Work out the finished part from the listing and answer in its coordinate system (mm). A direction names the side the tool comes from. Coordinates: 2 decimals unless noted, no trailing zeros. Order: outer loops, then holes, each group sorted by start corner. A loop starts at its lowest first (then second) coordinate and runs counter-clockwise, first axis right, second up. Notation, with made-up numbers: (58, -40) - (89, -40) arc R21 cw to (89, -13) - close; hole circle Ø2 at (18, 67.5). An arc over 180 degrees is marked (long way). Answer as a JSON object with one key per item and string values. Group by question number.
1) A tool of negligible diameter and unlimited length cuts with its end or side. For faces 1 (the face through (-33, -17, 10)), 2 (the face through (0, 22, 10)), 3 (the face through (-36, -22, 10)), 4 (the face through (-47.5, 0, 10)), from which of +Z, -Z, +X, -X, +Y, -Y can it reach the whole face along a straight path? Write none if from no direction.
2) Section A-A (x = 53.8) is taken. Give the vertices of the cut face in (y, z).
3) The mould has two halves that part along Y. Classify faces 5 (the face through (13.5, 31.07, 2.54)), 6 (the face through (59, -35, 3)), 7 (the face through (-61, 0, 2)): released by +Y, released by -Y, zero draft, split by the parting line, or undercut.
4) Section D-D (x = -34) is taken. Give the vertices of the cut face in (y, z).
5) Each of these flat-tipped pins is pushed along its axis until it touches: P1, Ø4, axis at x = -15, y = 31, coming from the +Z side; P2, Ø6, axis at x = 45, z = 13, coming from the +Y side; P3, Ø8, axis at x = -33, z = 10, coming from the -Y side. Where does it stop, or does it pass through?
6) Find the intervals of material crossed by line 1 along Y through (x, z) = (-53.8, 2.7); line 2 along Y through (x, z) = (-17, 11.25); line 3 along Y through (x, z) = (-31, 6.5), in increasing order.
7) Section C-C (y = 12) is taken. Give the vertices of the cut face in (x, z).
8) Section B-B (x = -15) is taken. Give the vertices of the cut face in (y, z).
from build123d import *

# Parameters (mm, degrees)
SKETCH_1_W          = 122
SKETCH_1_H          = 72
EXTRUDE_1_DEPTH     = 5
SKETCH_4_R          = 1.5
CUT_EXTRUDE_2_DEPTH = 10
SKETCH_5_W          = 5
SKETCH_5_H          = 5
EXTRUDE_3_DEPTH     = 10
SKETCH_6_R          = 1.5
CUT_EXTRUDE_3_DEPTH = 15
CUT_EXTRUDE_4_DEPTH = 25
FILLET_1_R          = 4
FILLET_3_R          = 5


with BuildPart() as part:
    # 草图1 → 凸台-拉伸1 (new body)
    with BuildSketch(Plane.XY):
        Rectangle(SKETCH_1_W, SKETCH_1_H)
    extrude(amount=EXTRUDE_1_DEPTH)

    # 草图4 → 切除-拉伸2 (cut)
    with BuildSketch(Plane.XY.offset(5)):
        with Locations((-53.8, 12)):
            Circle(SKETCH_4_R)
        with Locations((53.8, 12)):
            Circle(SKETCH_4_R)
        with Locations((53.8, -12)):
            Circle(SKETCH_4_R)
        with Locations(Location((-53.8, -12, 0), (0, 0, 180))):
            Circle(SKETCH_4_R)
    extrude(amount=-CUT_EXTRUDE_2_DEPTH, mode=Mode.SUBTRACT)

    # 草图5 → 凸台-拉伸3 (add)
    with BuildSketch(Plane.XY.offset(5)):
        Polygon((-42.5, 17), (42.5, 17), (42.5, 22), (-47.5, 22), (-47.5, -22), (-25, -22), (-25, -17), (-42.5, -17), align=None)
        with Locations((-22.5, -19.5)):
            Rectangle(SKETCH_5_W, SKETCH_5_H)
        Polygon((25, -36), (25, -31), (20, -31), (-20, -31), (-20, -22), (-25, -22), (-25, -36), align=None)
    extrude(amount=EXTRUDE_3_DEPTH)

    # 草图6 → 切除-拉伸3 (cut)
    with BuildSketch(Plane.XY.offset(5)):
        with Locations((0, 31)):
            Circle(SKETCH_6_R)
        with Locations((15, 31)):
            Circle(SKETCH_6_R)
        with Locations((30, 31)):
            Circle(SKETCH_6_R)
        with Locations((-15, 31)):
            Circle(SKETCH_6_R)
        with Locations((-30, 31)):
            Circle(SKETCH_6_R)
    extrude(amount=-CUT_EXTRUDE_3_DEPTH, mode=Mode.SUBTRACT)

    # 草图7 → 切除-拉伸4 (cut)
    with BuildSketch(Plane.XY.offset(5)):
        with BuildLine():
            ThreePointArc((44.8, 31.8), (43.3, 33.3), (41.8, 31.8))
            Line((41.8, 31.8), (43.3, 31.8))
            Line((43.3, 31.8), (43.3, 30.3))
            ThreePointArc((43.3, 30.3), (44.360660172, 30.739339828), (44.8, 31.8))
        make_face()
        with BuildLine():
            Line((43.3, 31.8), (41.8, 31.8))
            ThreePointArc((41.8, 31.8), (42.239339828, 30.739339828), (43.3, 30.3))
            Line((43.3, 30.3), (43.3, 31.8))
        make_face()
        with BuildLine():
            ThreePointArc((44.8, -31.8), (44.360660172, -30.739339828), (43.3, -30.3))
            Line((43.3, -30.3), (43.3, -31.8))
            Line((43.3, -31.8), (41.8, -31.8))
            ThreePointArc((41.8, -31.8), (43.3, -33.3), (44.8, -31.8))
        make_face()
        with BuildLine():
            Line((43.3, -31.8), (43.3, -30.3))
            ThreePointArc((43.3, -30.3), (42.239339828, -30.739339828), (41.8, -31.8))
            Line((41.8, -31.8), (43.3, -31.8))
        make_face()
        with BuildLine():
            ThreePointArc((-41.8, -31.8), (-42.239339828, -30.739339828), (-43.3, -30.3))
            Line((-43.3, -30.3), (-43.3, -31.8))
            Line((-43.3, -31.8), (-41.8, -31.8))
        make_face()
        with BuildLine():
            Line((-43.3, -31.8), (-43.3, -30.3))
            ThreePointArc((-43.3, -30.3), (-44.360660172, -32.860660172), (-41.8, -31.8))
            Line((-41.8, -31.8), (-43.3, -31.8))
        make_face()
        with BuildLine():
            Line((-43.3, 30.3), (-43.3, 31.8))
            Line((-43.3, 31.8), (-41.8, 31.8))
            ThreePointArc((-41.8, 31.8), (-44.360660172, 32.860660172), (-43.3, 30.3))
        make_face()
        with BuildLine():
            Line((-41.8, 31.8), (-43.3, 31.8))
            Line((-43.3, 31.8), (-43.3, 30.3))
            ThreePointArc((-43.3, 30.3), (-42.239339828, 30.739339828), (-41.8, 31.8))
        make_face()
    extrude(amount=-CUT_EXTRUDE_4_DEPTH, mode=Mode.SUBTRACT)

    # 圆角1
    fillet_1_edges = [part.edges().sort_by_distance(p)[0] for p in [
        (-47.5, 22, 10),
        (-47.5, -22, 10),
        (-25, -22, 10),
        (-25, -36, 10),
        (-20, -17, 10),
    ]]
    fillet(fillet_1_edges, radius=FILLET_1_R)

    # 圆角3
    fillet_3_edges = [part.edges().sort_by_distance(p)[0] for p in [
        (61, -36, 2.5),
        (-61, -36, 2.5),
        (-61, 36, 2.5),
        (61, 36, 2.5),
    ]]
    fillet(fillet_3_edges, radius=FILLET_3_R)


solid = part.part
Report:
{
 "1": {"face 1": "+Z, +X", "face 2": "+Z, +X, -X, +Y", "face 3": "+Z, -X, -Y", "face 4": "+Z, -X, +Y, -Y"},
 "2": {"outline": "(-36, 0) - (-13.5, 0) - (-13.5, 5) - (-36, 5) - close; (-10.5, 0) - (10.5, 0) - (10.5, 5) - (-10.5, 5) - close; (13.5, 0) - (36, 0) - (36, 5) - (13.5, 5) - close"},
 "3": {"face 5": "undercut", "face 6": "released by -Y", "face 7": "zero draft"},
 "4": {"outline": "(-36, 0) - (36, 0) - (36, 5) - (22, 5) - (22, 15) - (17, 15) - (17, 5) - (-17, 5) - (-17, 15) - (-22, 15) - (-22, 5) - (-36, 5) - close"},
 "5": {"P1": "stops at z = 5", "P2": "stops at y = 22", "P3": "stops at y = -22"},
 "6": {"line 1": "y = -36 to -13.5, -10.5 to 10.5, 13.5 to 36", "line 2": "y = -36 to -31, 17 to 22", "line 3": "y = -22 to -17, 17 to 22"},
 "7": {"outline": "(-61, 0) - (-55.3, 0) - (-55.3, 5) - (-61, 5) - close; (-52.3, 0) - (52.3, 0) - (52.3, 5) - (-42.5, 5) - (-42.5, 15) - (-47.5, 15) - (-47.5, 5) - (-52.3, 5) - close; (55.3, 0) - (61, 0) - (61, 5) - (55.3, 5) - close"},
 "8": {"outline": "(-36, 0) - (29.5, 0) - (29.5, 5) - (22, 5) - (22, 15) - (17, 15) - (17, 5) - (-31, 5) - (-31, 15) - (-36, 15) - close; (32.5, 0) - (36, 0) - (36, 5) - (32.5, 5) - close"}
}
